from build123d import *

# Parameters (mm, degrees)
SKETCH_1_R          = 39
SKETCH_1_R_2        = 30
EXTRUDE_1_DEPTH     = 10
SKETCH_2_R          = 36
SKETCH_2_R_2        = 33
CUT_EXTRUDE_1_DEPTH = 1
CUT_EXTRUDE_START   = -1
SKETCH_3_R          = 36
SKETCH_3_R_2        = 33
CUT_EXTRUDE_2_DEPTH = 1


with BuildPart() as part:
    # 草图1 → 凸台-拉伸1 (new body)
    with BuildSketch(Plane(origin=(0, 0, 0), x_dir=(0, 0, -1), z_dir=(1, 0, 0))):
        Circle(SKETCH_1_R)
        Circle(SKETCH_1_R_2, mode=Mode.SUBTRACT)
    extrude(amount=EXTRUDE_1_DEPTH)

    # 草图2 → 切除-拉伸1 (cut)
    with BuildSketch(Plane(origin=(10, 0, 0), x_dir=(0, 0, -1), z_dir=(1, 0, 0))):
        Circle(SKETCH_2_R)
        Circle(SKETCH_2_R_2, mode=Mode.SUBTRACT)
    extrude(amount=-CUT_EXTRUDE_1_DEPTH, mode=Mode.SUBTRACT)

    # 草图3 → 切除-拉伸2 (cut)
    with BuildSketch(Plane.ZY.offset(CUT_EXTRUDE_START)):
        with Locations(Location((0, 0, 0), (0, 0, 180))):
            Circle(SKETCH_3_R)
        with Locations(Location((0, 0, 0), (0, 0, 180))):
            Circle(SKETCH_3_R_2, mode=Mode.SUBTRACT)
    extrude(amount=CUT_EXTRUDE_2_DEPTH, mode=Mode.SUBTRACT)


solid = part.part
Could you check a few things on this model? Use its own coordinates, in mm. A direction names the side the tool comes from. Coordinates: 2 decimals unless noted, no trailing zeros. Order: outer loops, then holes, each group sorted by start corner. A loop starts at its lowest first (then second) coordinate and runs counter-clockwise, first axis right, second up. Notation, with made-up numbers: (9, 53.5) - (47, 53.5) arc R32 cw to (47, 85.5) - close; hole circle Ø8 at (45.25, -33.5). An arc over 180 degrees is marked (long way). Answer in a Markdown table with one row per item. Add a question column.
(1) If we mould it in two halves opening along Z, with no side actions, what happens to faces 4 (the face through (0, -34.5, -11.4)), 5 (the face through (4.93, 38.668, 5.077)), 6 (the face through (9.507, 35.694, 4.686))? For each: released by +Z, released by -Z, zero draft, split by the parting line, or undercut.
(2) On a 3-axis mill with a long thin cutter (end or side, diameter ignored), from which of +Z, -Z, +X, -X, +Y, -Y can I reach the whole of each face in a straight line? I mean faces 1 (the face through (10, -27, -15)), 2 (the face through (0.507, -9.912, -31.476)), 3 (the face through (9, -29.2, -15.8)). Say none if no direction works.
(3) If we section it at A-A, the plane z = 0: Please give me the cut outline in (x, y), then the cut area to 3 significant figures.
(4) If we section it at C-C, the plane x = 5: Please give me the cut outline in (y, z), then the cut area to 3 significant figures.
(5) I need wall thicknesses on L1, parallel to Y at x = 0.25, z = 0; L2, parallel to Y at x = 0.5, z = 15.5; L3, parallel to X at y = 15, z = 32. Which ranges of each line are inside material? Lowest first, please.
(6) Will these pins go through, and if not, where does the flat tip stop? pin 1 (1.5 mm diameter, centred on x = 4.5, y = 15.5, fed in from +Z); pin 2 (5 mm diameter, centred on x = 7, z = 21.5, fed in from +Y).
Results are:
| question | item | result |
|---|---|---|
| 1 | face 4 | zero draft |
| 1 | face 5 | split by the parting line |
| 1 | face 6 | undercut |
| 2 | face 1 | +Z, -Z, +X, +Y, -Y |
| 2 | face 2 | -X |
| 2 | face 3 | +X |
| 3 | outline | (0, -39) - (10, -39) - (10, -36) - (9, -36) - (9, -33) - (10, -33) - (10, -30) - (0, -30) - (0, -33) - (1, -33) - (1, -36) - (0, -36) - close; (0, 30) - (10, 30) - (10, 33) - (9, 33) - (9, 36) - (10, 36) - (10, 39) - (0, 39) - (0, 36) - (1, 36) - (1, 33) - (0, 33) - close |
| 3 | area | 168 mm2 |
| 4 | outline | circle Ø78 at (0, 0); hole circle Ø60 at (0, 0) |
| 4 | area | 1,950 mm2 |
| 5 | L1 | y = -39 to -36, -33 to -30, 30 to 33, 36 to 39 |
| 5 | L2 | y = -35.79 to -32.49, -29.13 to -25.69, 25.69 to 29.13, 32.49 to 35.79 |
| 5 | L3 | x = 1 to 9 |
| 6 | pin 1 | stops at z = 36.1 |
| 6 | pin 2 | stops at y = 34.06 |
